Geometry: final body of the model. Coordinates: model frame, mm. A direction names the side the tool comes from. Round coordinates to 2 decimals unless told otherwise and drop trailing zeros. Write each loop counter-clockwise with the first axis right and the second up, starting at its lowest first coordinate (ties: lowest second). Pieces come first, ordered by that corner, then holes. Notation, with made-up numbers: (34, 47) -> (74, 47) arc R16 cw to (74, 74) -> close; hole circle Ø4 at (-12, 24). An arc over 180 degrees is marked (long way). Use one line per item in the form item = value. Start each with the question number.
1. Line query: L1, parallel to Y at x = -28.5, z = 8; L2, parallel to X at y = -50.5, z = 6; L3, parallel to Y at x = 16.5, z = 7.5. Output: solid intervals per line, ascending.
2. Cut plane B-B, the plane x = 6. Return the cut outline in (y, z).
3. Pin query (flat end, axial travel): pin 1 Ø3.5 at (x, z) = (16, 22.5) entering from +Y; pin 2 Ø1.9 at (x, z) = (-57.5, 16) entering from +Y; pin 3 Ø1.5 at (x, y) = (-30, -21) entering from -Z. Return the tip coordinate at first contact, or that it passes through.
4. Reachability of faces 1 (the face through (-3.5, -56, 18)), 2 (the face through (-60, -20, 15)) from +Z, -Z, +X, -X, +Y, -Y: full face, straight path, thin tool, end or side. Return the list, or none.
5. Draft query along X for faces 3 (the face through (-55.94, 16.08, 13.46)), 4 (the face through (-57.15, -56.99, 14.8)), 5 (the face through (20, -20, 15)). Return one class per face: pulls with the +X half, pulls with the -X half, needs draft (parallel to the pull), parting line crosses it, or undercut.
6. Cut plane A-A, the plane y = 8. Return the cut outline in (x, z), plus the area to 3 significant figures.
```python
from build123d import *

# Parameters (mm, degrees)
F1_DEPTH    = 30
F2_T        = -1.5
F3_W        = 1.5
F3_H        = 4.25
F3_W_2      = 4.25
F3_H_2      = 1.5
F4_DEPTH    = 22
F5_SIZE     = 1.2
F6_R        = 1
F7_W        = 2
F7_H        = 60
F8_DEPTH    = 30.001
F10_SIZE2   = 2
F10_SIZE    = 5
F10_2_SIZE2 = 2
F10_2_SIZE  = 5
F10_3_SIZE2 = 2
F10_3_SIZE  = 5
F10_4_SIZE2 = 2
F10_4_SIZE  = 5
F10_5_SIZE2 = 2
F10_5_SIZE  = 5
F10_6_SIZE2 = 2
F10_6_SIZE  = 5
F10_7_SIZE2 = 2
F10_7_SIZE  = 5
F10_8_SIZE2 = 2
F10_8_SIZE  = 5


# Not quite as in the source:
# - a pattern or mirror of a feature is missing from the dataset's text; its kind, count and spacing are read off the source's solid


with BuildPart() as f1:
    # F0 (on Top) → F1 (new body)
    with BuildSketch(Plane.XY):
        with BuildLine():
            ThreePointArc((20, 10), (17.0710678119, 17.0710678119), (10, 20))
            Line((10, 20), (-50, 20))
            ThreePointArc((-50, 20), (-57.0710678119, 17.0710678119), (-60, 10))
            Line((-60, 10), (-60, -50))
            ThreePointArc((-60, -50), (-57.0710678119, -57.0710678119), (-50, -60))
            Line((-50, -60), (10, -60))
            ThreePointArc((10, -60), (17.0710678119, -57.0710678119), (20, -50))
            Line((20, -50), (20, 10))
        make_face()
    extrude(amount=F1_DEPTH)

    # F2
    f2_openings = [f1.faces().sort_by_distance(p)[0] for p in [
        (-20, -20, 0),
    ]]
    offset(amount=F2_T, openings=f2_openings)

    # F3 (on face) → F4 (join)
    with BuildSketch(Plane(origin=(0, 0, 28.5), x_dir=(1, 0, 0), z_dir=(0, 0, -1))):
        with Locations((-35.75, 56.375)):
            Rectangle(F3_W, F3_H)
        with Locations((-4.25, 56.375)):
            Rectangle(F3_W, F3_H)
        with Locations((-56.875, 4.25)):
            Rectangle(F3_W_2, F3_H_2)
        with Locations((-56.875, 35.75)):
            Rectangle(F3_W_2, F3_H_2)
        with Locations((-4.75, -16.875)):
            Rectangle(F3_W, F3_H)
        with Locations((-36.25, -16.875)):
            Rectangle(F3_W, F3_H)
        with Locations((16.375, 35.25)):
            Rectangle(F3_W_2, F3_H_2)
        with Locations((16.375, 3.75)):
            Rectangle(F3_W_2, F3_H_2)
    extrude(amount=F4_DEPTH)

    # F5
    f5_edges = [f1.edges().sort_by_distance(p)[0] for p in [
        (3, 18.5, 28.5),
        (-20.5, 18.5, 28.5),
        (-43.5, 18.5, 28.5),
        (18.5, -19.5, 28.5),
        (18.5, -43, 28.5),
        (-58.5, -20, 28.5),
        (-58.5, -43.25, 28.5),
        (-20, -58.5, 28.5),
        (16.010408, 16.010408, 28.5),
        (18.5, 3.5, 28.5),
        (16.010408, -56.010408, 28.5),
        (3.25, -58.5, 28.5),
        (-43.25, -58.5, 28.5),
        (-56.010408, -56.010408, 28.5),
        (-58.5, 3.25, 28.5),
        (-56.010408, 16.010408, 28.5),
    ]]
    chamfer(f5_edges, length=F5_SIZE)

    # F6
    f6_edges = [f1.edges().sort_by_distance(p)[0] for p in [
        (20, -20, 30),
        (20, -20, 0),
        (17.071068, 17.071068, 0),
        (-20, 20, 0),
        (-57.071068, 17.071068, 0),
        (-60, -20, 0),
        (-57.071068, -57.071068, 0),
        (-20, -60, 0),
        (17.071068, -57.071068, 0),
        (17.071068, 17.071068, 30),
        (-20, 20, 30),
        (-57.071068, 17.071068, 30),
        (-60, -20, 30),
        (-57.071068, -57.071068, 30),
        (-20, -60, 30),
        (17.071068, -57.071068, 30),
    ]]
    fillet(f6_edges, radius=F6_R)

    # F7 (on face) → F8 (cut, through all)
    with BuildSketch(Plane.XY.offset(30)):
        with Locations((-51, -20)):
            Rectangle(F7_W, F7_H)
    f8 = extrude(amount=-F8_DEPTH, mode=Mode.SUBTRACT)

    # F8_copies: F8 across plane
    add(f8.mirror(Plane(origin=(-20, 0, 0), x_dir=(0, 0, 1), z_dir=(1, 0, 0))), mode=Mode.SUBTRACT)

    # F10
    f10_edges = [f1.edges().sort_by_distance(p)[0] for p in [
        (-54.75, -4.25, 6.5),
    ]]
    f10_side = f1.faces().sort_by_distance((-54.75, -4.25, 17.5))[0]
    chamfer(f10_edges, length=F10_SIZE, length2=F10_SIZE2, reference=f10_side)

    # F10#2
    f10_2_edges = [f1.edges().sort_by_distance(p)[0] for p in [
        (-54.75, -35.75, 6.5),
    ]]
    f10_2_side = f1.faces().sort_by_distance((-54.75, -35.75, 17.5))[0]
    chamfer(f10_2_edges, length=F10_2_SIZE, length2=F10_2_SIZE2, reference=f10_2_side)

    # F10#3
    f10_3_edges = [f1.edges().sort_by_distance(p)[0] for p in [
        (-35.75, -54.25, 6.5),
    ]]
    f10_3_side = f1.faces().sort_by_distance((-35.75, -54.25, 17.5))[0]
    chamfer(f10_3_edges, length=F10_3_SIZE, length2=F10_3_SIZE2, reference=f10_3_side)

    # F10#4
    f10_4_edges = [f1.edges().sort_by_distance(p)[0] for p in [
        (-4.25, -54.25, 6.5),
    ]]
    f10_4_side = f1.faces().sort_by_distance((-4.25, -54.25, 17.5))[0]
    chamfer(f10_4_edges, length=F10_4_SIZE, length2=F10_4_SIZE2, reference=f10_4_side)

    # F10#5
    f10_5_edges = [f1.edges().sort_by_distance(p)[0] for p in [
        (14.25, -35.25, 6.5),
    ]]
    f10_5_side = f1.faces().sort_by_distance((14.25, -35.25, 17.5))[0]
    chamfer(f10_5_edges, length=F10_5_SIZE, length2=F10_5_SIZE2, reference=f10_5_side)

    # F10#6
    f10_6_edges = [f1.edges().sort_by_distance(p)[0] for p in [
        (14.25, -3.75, 6.5),
    ]]
    f10_6_side = f1.faces().sort_by_distance((14.25, -3.75, 17.5))[0]
    chamfer(f10_6_edges, length=F10_6_SIZE, length2=F10_6_SIZE2, reference=f10_6_side)

    # F10#7
    f10_7_edges = [f1.edges().sort_by_distance(p)[0] for p in [
        (-4.75, 14.75, 6.5),
    ]]
    f10_7_side = f1.faces().sort_by_distance((-4.75, 14.75, 17.5))[0]
    chamfer(f10_7_edges, length=F10_7_SIZE, length2=F10_7_SIZE2, reference=f10_7_side)

    # F10#8
    f10_8_edges = [f1.edges().sort_by_distance(p)[0] for p in [
        (-36.25, 14.75, 6.5),
    ]]
    f10_8_side = f1.faces().sort_by_distance((-36.25, 14.75, 17.5))[0]
    chamfer(f10_8_edges, length=F10_8_SIZE, length2=F10_8_SIZE2, reference=f10_8_side)


solid = f1.part
```
Outcome:
q1.L1 = -60 to -58.5, 18.5 to 20
q1.L2 = -59.99 to -58.49, 18.49 to 19.99
q1.L3 = -57.6 to -55.48, -36 to -34.5, -4.5 to -3, 15.48 to 17.6
q2.outline = (-60, 1) arc R1 ccw to (-59, 0) -> (-58.5, 0) -> (-58.5, 27.3) -> (-57.3, 28.5) -> (17.3, 28.5) -> (18.5, 27.3) -> (18.5, 0) -> (19, 0) arc R1 ccw to (20, 1) -> (20, 29) arc R1 ccw to (19, 30) -> (-59, 30) arc R1 ccw to (-60, 29) -> close
q3.pin_1 = 19.05
q3.pin_2 = 17.56
q3.pin_3 = 28.5
q4.face_1 = -Z
q4.face_2 = +Z, -Z, -X, +Y, -Y
q5.face_3 = undercut
q5.face_4 = pulls with the -X half
q5.face_5 = pulls with the +X half
q6.outline = (-60, 1) arc R1 ccw to (-59, 0) -> (-58.5, 0) -> (-58.5, 27.3) -> (-57.3, 28.5) -> (-52, 28.5) -> (-52, 30) -> (-59, 30) arc R1 ccw to (-60, 29) -> close; (-50, 28.5) -> (10, 28.5) -> (10, 30) -> (-50, 30) -> close; (12, 28.5) -> (17.3, 28.5) -> (18.5, 27.3) -> (18.5, 0) -> (19, 0) arc R1 ccw to (20, 1) -> (20, 29) arc R1 ccw to (19, 30) -> (12, 30) -> close
q6.area = 200 mm^2
